Read the model definition and answer for the solid it produces. Units are mm, in the model's axes. A direction names the side the tool comes from. Give positions to 0.01 mm unless a question says otherwise; leave off trailing zeros. Write each loop counter-clockwise with the first axis right and the second up, starting at its lowest first coordinate (ties: lowest second). Pieces come first, ordered by that corner, then holes. Notation, with made-up numbers: (-10, 28.5) -> (12, 28.5) arc R14 ccw to (12, 54.5) -> close; hole circle Ø10 at (-28.75, 10.25). An arc over 180 degrees is marked (long way). Use a Markdown table: item, result.
from build123d import *

# Parameters (mm, degrees)
SKETCH2_R               = 3.175
BOSS_EXTRUDE1_DEPTH     = 6.096
SKETCH3_R               = 5.588
BOSS_EXTRUDE2_DEPTH     = 1.27
SKETCH4_R               = 5.08
BOSS_EXTRUDE3_DEPTH     = 4.064
SKETCH5_R               = 4.445
BOSS_EXTRUDE4_DEPTH     = 4.699
SKETCH6_R               = 3.3655
CUT_EXTRUDE1_DEPTH      = 7.112
SKETCH7_R               = 2.2225
CUT_EXTRUDE2_DEPTH      = 8.255
SKETCH8_R               = 0.6985
CUT_EXTRUDE3_DEPTH      = 18.960961249
CUT_EXTRUDE4_DEPTH      = 8.255
CUT_EXTRUDE4_DEPTH_BACK = 8.255
SKETCH9_R               = 0.6985


with BuildPart() as part:
    # Sketch2 → Boss-Extrude1 (new body)
    with BuildSketch(Plane.XY):
        Circle(SKETCH2_R)
    extrude(amount=-BOSS_EXTRUDE1_DEPTH)

    # Sketch3 → Boss-Extrude2 (add)
    with BuildSketch(Plane(origin=(0, 0, -6.096), x_dir=(-1, 0, 0), z_dir=(0, 0, -1))):
        Circle(SKETCH3_R)
    extrude(amount=BOSS_EXTRUDE2_DEPTH)

    # Sketch4 → Boss-Extrude3 (add)
    with BuildSketch(Plane(origin=(0, 0, -7.366), x_dir=(-1, 0, 0), z_dir=(0, 0, -1))):
        Circle(SKETCH4_R)
    extrude(amount=BOSS_EXTRUDE3_DEPTH)

    # Sketch5 → Boss-Extrude4 (add)
    with BuildSketch(Plane(origin=(0, 0, -11.43), x_dir=(-1, 0, 0), z_dir=(0, 0, -1))):
        Circle(SKETCH5_R)
    extrude(amount=BOSS_EXTRUDE4_DEPTH)

    # Sketch6 → Cut-Extrude1 (cut)
    with BuildSketch(Plane(origin=(0, 0, -16.129), x_dir=(-1, 0, 0), z_dir=(0, 0, -1))):
        Circle(SKETCH6_R)
    extrude(amount=-CUT_EXTRUDE1_DEPTH, mode=Mode.SUBTRACT)

    # Sketch7 → Cut-Extrude2 (cut)
    with BuildSketch(Plane(origin=(0, 0, -9.017), x_dir=(-1, 0, 0), z_dir=(0, 0, -1))):
        Circle(SKETCH7_R)
    extrude(amount=-CUT_EXTRUDE2_DEPTH, mode=Mode.SUBTRACT)

    # Sketch8 → Cut-Extrude3 (cut, through all)
    with BuildSketch(Plane.XY):
        Circle(SKETCH8_R)
    extrude(amount=-CUT_EXTRUDE3_DEPTH, mode=Mode.SUBTRACT)

    # Sketch9 → Cut-Extrude4 (cut, two sides: drawn at the far end of the back side and taken through both)
    with BuildSketch(Plane(origin=(0, 0, 0), x_dir=(1, 0, 0), z_dir=(0, 1, 0)).offset(-CUT_EXTRUDE4_DEPTH_BACK)):
        with Locations(Location((0, 10.549993494, 0), (0, 0, 90))):
            Circle(SKETCH9_R)
    extrude(amount=CUT_EXTRUDE4_DEPTH + CUT_EXTRUDE4_DEPTH_BACK, mode=Mode.SUBTRACT)


solid = part.part
Item 1: A tool of negligible diameter and unlimited length cuts with its end or side. For faces 1 (the face through (-0.69, -3.1, -3.01)), 2 (the face through (0.73, -3.285, -12.623)), 3 (the face through (0, 1, 0)), from which of +Z, -Z, +X, -X, +Y, -Y can it reach the whole face along a straight path? Write none if from no direction.
Return value:
| item | result |
|---|---|
| face 1 | +Z |
| face 2 | -Z |
| face 3 | +Z, +X, -X, +Y, -Y |
Item 2: Each of these flat-tipped pins is pushed along its axis until it touches: P1, Ø1.5, axis at x = 2.5, z = -7, coming from the -Y side; P2, Ø6, axis at x = 0, y = 0, coming from the -Z side; P3, Ø2, axis at y = -3.5, z = -3, coming from the +X side. Where does it stop, or does it pass through?
Return value:
| item | result |
|---|---|
| P1 | y = -5.31 |
| P2 | z = -9.02 |
| P3 | x = 1.96 |
Item 3: For a pull along X with two mould halves and no side action, classify faces 4 (the face through (0.43, -4.2, -10)), 5 (the face through (4.434, -3.4, -6.722)), 6 (the face through (-2, 3, -16.129)) as +X half, -X half, draft (parallel to the pull), parting line (faces both ways), or undercut.
Return value:
| item | result |
|---|---|
| face 4 | undercut |
| face 5 | parting line |
| face 6 | draft |
Item 4: A cutting plane is placed at A-A (y = 0). Give the vertices of the cut face in (x, z) (1 decimal), then the cut area to 3 significant figures.
Return value:
| item | result |
|---|---|
| outline | (-5.6, -7.4) -> (-5.1, -7.4) -> (-5.1, -11.4) -> (-4.4, -11.4) -> (-4.4, -16.1) -> (-3.4, -16.1) -> (-3.4, -9) -> (-2.2, -9) -> (-2.2, -0.8) -> (-0.7, -0.8) -> (-0.7, 0) -> (-3.2, 0) -> (-3.2, -6.1) -> (-5.6, -6.1) -> close; (0.7, -0.8) -> (2.2, -0.8) -> (2.2, -9) -> (3.4, -9) -> (3.4, -16.1) -> (4.4, -16.1) -> (4.4, -11.4) -> (5.1, -11.4) -> (5.1, -7.4) -> (5.6, -7.4) -> (5.6, -6.1) -> (3.2, -6.1) -> (3.2, 0) -> (0.7, 0) -> close |
| area | 50.3 mm^2 |
Item 5: A cutting plane is placed at B-B (z = -10.5). Give the vertices of the cut face in (x, y).
Return value:
| item | result |
|---|---|
| outline | (-0.7, -5.03) -> (-0.7, -3.29) arc R3.37 cw to (-0.7, 3.29) -> (-0.7, 5.03) arc R5.08 ccw to start; (0.7, -5.03) arc R5.08 ccw to (0.7, 5.03) -> (0.7, 3.29) arc R3.37 cw to (0.7, -3.29) -> close |
Item 6: Straight lines are drawn through the part: line 1 along Y through (x, z) = (0, -13.25) (1 decimal); line 2 along Y through (x, z) = (0, -0.2) (1 decimal); line 3 along Z through (x, y) = (4.75, 2). For each, find the intervals that lie inside material, in ascending order. Write a range as [from, to].
Return value:
| item | result |
|---|---|
| line 1 | [-4.4, -3.4], [3.4, 4.4] |
| line 2 | [-3.2, -0.7], [0.7, 3.2] |
| line 3 | [-7.37, -6.1] |
Item 7: A cutting plane is placed at D-D (x = 2). Give the vertices of the cut face in (y, z), then the cut area to 3 significant figures.
Return value:
| item | result |
|---|---|
| outline | (-5.22, -7.37) -> (-4.67, -7.37) -> (-4.67, -11.43) -> (-3.97, -11.43) -> (-3.97, -16.13) -> (-2.71, -16.13) -> (-2.71, -9.02) -> (-0.97, -9.02) -> (-0.97, -0.76) -> (0.97, -0.76) -> (0.97, -9.02) -> (2.71, -9.02) -> (2.71, -16.13) -> (3.97, -16.13) -> (3.97, -11.43) -> (4.67, -11.43) -> (4.67, -7.37) -> (5.22, -7.37) -> (5.22, -6.1) -> (2.47, -6.1) -> (2.47, 0) -> (-2.47, 0) -> (-2.47, -6.1) -> (-5.22, -6.1) -> close |
| area | 64.1 mm^2 |
Item 8: A cutting plane is placed at C-C (x = 0). Count the separate pieces of the cut face and the enclosed holes in it, then the cut area to 3 significant figures.
Return value:
| item | result |
|---|---|
| separate pieces | 4 |
| enclosed holes | 0 |
| area | 45.5 mm^2 |
